Read the model definition and answer for the solid it produces. Units are mm, in the model's axes. A direction names the side the tool comes from. Coordinates: 2 decimals unless noted, no trailing zeros. Write each loop counter-clockwise with the first axis right and the second up, starting at its lowest first coordinate (ties: lowest second). Pieces come first, ordered by that corner, then holes.
(1) Straight lines are drawn through the part: line 1 along Z through (x, y) = (-3.5, -1.25); line 2 along X through (y, z) = (-0.5, -59); line 3 along Y through (x, z) = (-0.25, -70). For each, find the intervals that lie inside material, in ascending order.
(2) Which of the six approach directions +Z, -Z, +X, -X, +Y, -Y give full straight-line access (tool end or side, diameter ignored) to faces 1 (the flat face through (2.2, -3.3, 62)), 2 (the cylindrical face through (-5, 0, -48))?
(3) Given pin 1 (1 mm diameter, centred on y = 3, z = -41, fed in from -X); pin 2 (1.5 mm diameter, centred on y = -2.5, z = -34.5, fed in from +X); pin 3 (3 mm diameter, centred on y = 3.5, z = -48.5, fed in from -X), each flat-ended and moving along its own axis, determine where each tip first touches the part or whether it passes through.
(4) Determine the mould class of faces 3 (the flat face through (0, 0, 152)), 4 (the flat face through (2.2, -3.3, 60)), 5 (the cylindrical face through (-1.08, -4.88, 29.58)) for opening direction Z: pulls with the +Z half, pulls with the -Z half, needs draft (parallel to the pull), parting line crosses it, or undercut.
(5) The part is cut by section A-A, the plane x = 2. Determine the outline of the cut face in (y, z), and give its area (3 significant figures).
(6) The part is cut by section B-B, the plane z = 76.5. Determine the outline of the cut face in (x, y), and give its area (3 significant figures).
```python
from build123d import *

# Parameters (mm, degrees)
SKETCH_1_R      = 5
EXTRUDE_1_DEPTH = 60
SKETCH_2_R      = 3.5
EXTRUDE_2_DEPTH = 2
EXTRUDE_START   = 2
SKETCH_3_R      = 3.5
EXTRUDE_3_DEPTH = 2
EXTRUDE_START_2 = 90
SKETCH_4_R      = 5
EXTRUDE_4_DEPTH = 90
SKETCH_5_R      = 5
EXTRUDE_5_DEPTH = 90


with BuildPart() as part:
    # 草图1 → 凸台-拉伸1 (new body)
    with BuildSketch(Plane.XY):
        Circle(SKETCH_1_R)
    extrude(amount=EXTRUDE_1_DEPTH)

    # 草图2 → 凸台-拉伸2 (add)
    with BuildSketch(Plane.XY.offset(60)):
        Circle(SKETCH_2_R)
    extrude(amount=EXTRUDE_2_DEPTH)

    # 草图3 → 凸台-拉伸3 (add)
    with BuildSketch(Plane(origin=(0, 0, 0), x_dir=(-1, 0, 0), z_dir=(0, 0, -1)).offset(EXTRUDE_START)):
        with Locations(Location((0, 0, 0), (0, 0, 180))):
            Circle(SKETCH_3_R)
    extrude(amount=-EXTRUDE_3_DEPTH)

    # 草图4 → 凸台-拉伸4 (add)
    with BuildSketch(Plane(origin=(0, 0, -2), x_dir=(-1, 0, 0), z_dir=(0, 0, -1)).offset(EXTRUDE_START_2)):
        with Locations(Location((0, 0, 0), (0, 0, 180))):
            Circle(SKETCH_4_R)
    extrude(amount=-EXTRUDE_4_DEPTH)

    # 草图5 → 凸台-拉伸5 (add)
    with BuildSketch(Plane.XY.offset(62)):
        Circle(SKETCH_5_R)
    extrude(amount=EXTRUDE_5_DEPTH)


solid = part.part
```
Computed:
1. line 1: z = -92 to -2, 0 to 60, 62 to 152
1. line 2: x = -4.97 to 4.97
1. line 3: y = -4.99 to 4.99
2. face 1: none
2. face 2: +Z, -Z
3. pin 1: stops at x = -4.33
3. pin 2: stops at x = 4.68
3. pin 3: stops at x = -4.58
4. face 3: pulls with the +Z half
4. face 4: undercut
4. face 5: needs draft
5. outline: (-4.58, -92) - (4.58, -92) - (4.58, -2) - (2.87, -2) - (2.87, 0) - (4.58, 0) - (4.58, 60) - (2.87, 60) - (2.87, 62) - (4.58, 62) - (4.58, 152) - (-4.58, 152) - (-4.58, 62) - (-2.87, 62) - (-2.87, 60) - (-4.58, 60) - (-4.58, 0) - (-2.87, 0) - (-2.87, -2) - (-4.58, -2) - close
5. area: 2,220 mm2
6. outline: circle Ø10 at (0, 0)
6. area: 78.5 mm2
